Can you work these out from the model? Positions are in its coordinate system, mm. A direction names the side the tool comes from. Round coordinates to 2 decimals unless told otherwise and drop trailing zeros. Loops run counter-clockwise (first coordinate to the right, second up) from the corner with the lowest first, then second, coordinate; pieces in that order, holes last. Notation, with made-up numbers: (-34, 26.5) -> (25, 26.5) arc R33 cw to (25, 62.5) -> close; hole circle Ø5 at (28, -38). An arc over 180 degrees is marked (long way). Answer as a JSON object with one key per item and string values.
```python
from build123d import *

# Parameters (mm, degrees)
SKETCH2_W           = 23
SKETCH2_H           = 32
SKETCH2_R           = 5.5
SKETCH2_R_2         = 20
SKETCH2_W_2         = 18
SKETCH2_H_2         = 25
BOSS_EXTRUDE1_DEPTH = 3
BOSS_EXTRUDE2_DEPTH = 3
SKETCH4_W           = 180
SKETCH4_H           = 158
BOSS_EXTRUDE3_DEPTH = 3
SKETCH6_W           = 1.5
SKETCH6_H           = 3
CUT_EXTRUDE4_DEPTH  = 177
SKETCH8_W           = 180
SKETCH8_H           = 147
BOSS_EXTRUDE5_DEPTH = 3
SKETCH9_R           = 5
SKETCH9_W           = 13.5
SKETCH9_H           = 6
CUT_EXTRUDE5_DEPTH  = 10


with BuildPart() as part:
    # Sketch2 → Boss-Extrude1 (new body)
    # profile 1 of 2: a face of its own
    with BuildSketch(Plane.XY):
        Polygon((90, 180), (0, 180), (0, 130), (0, 0), (90, 0), (90, 73), (47.5, 73), (47.5, 130), (90, 130), align=None)
        with Locations((36, 37)):
            Rectangle(SKETCH2_W, SKETCH2_H, mode=Mode.SUBTRACT)
        with Locations((22, 101.5)):
            Circle(SKETCH2_R, mode=Mode.SUBTRACT)
    # profile 2 of 2: a face of its own
    with BuildSketch(Plane.XY):
        Polygon((180, 180), (90, 180), (90, 130), (132.5, 130), (132.5, 73), (90, 73), (90, 0), (180, 0), align=None)
        with Locations((142, 37)):
            Circle(SKETCH2_R_2, mode=Mode.SUBTRACT)
        with Locations((161.5, 101.5)):
            Rectangle(SKETCH2_W_2, SKETCH2_H_2, mode=Mode.SUBTRACT)
    extrude(amount=-BOSS_EXTRUDE1_DEPTH)

    # Sketch3 → Boss-Extrude2 (add)
    with BuildSketch(Plane(origin=(0, 0, 0), x_dir=(0, 0, -1), z_dir=(1, 0, 0))):
        Polygon((158, 180), (3, 180), (3, 90), (3, 0), (50, 0), (158, 0), align=None)
    boss_extrude2 = extrude(amount=BOSS_EXTRUDE2_DEPTH)

    # Mirror1: Boss-Extrude2 across plane
    add(boss_extrude2.mirror(Plane(origin=(90, 0, 0), x_dir=(0, 0, 1), z_dir=(1, 0, 0))))

    # Sketch4 → Boss-Extrude3 (add)
    with BuildSketch(Plane(origin=(0, 0, 0), x_dir=(1, 0, 0), z_dir=(0, 1, 0))):
        with Locations((90, 79)):
            Rectangle(SKETCH4_W, SKETCH4_H)
    extrude(amount=BOSS_EXTRUDE3_DEPTH)

    # Sketch6 → Cut-Extrude4 (cut)
    with BuildSketch(Plane(origin=(0, 180, 0), x_dir=(1, 0, 0), z_dir=(0, 1, 0))):
        with Locations((2.25, 151.5)):
            Rectangle(SKETCH6_W, SKETCH6_H)
    cut_extrude4 = extrude(amount=-CUT_EXTRUDE4_DEPTH, mode=Mode.SUBTRACT)

    # Mirror2: Cut-Extrude4 across plane
    add(cut_extrude4.mirror(Plane(origin=(90, 0, 0), x_dir=(0, 0, 1), z_dir=(1, 0, 0))), mode=Mode.SUBTRACT)

    # Sketch8 → Boss-Extrude5 (add)
    with BuildSketch(Plane(origin=(0, 180, 0), x_dir=(1, 0, 0), z_dir=(0, 1, 0))):
        with Locations((90, 73.5)):
            Rectangle(SKETCH8_W, SKETCH8_H)
    extrude(amount=-BOSS_EXTRUDE5_DEPTH)

    # Sketch9 → Cut-Extrude5 (cut)
    with BuildSketch(Plane(origin=(180, 0, 0), x_dir=(0, 0, -1), z_dir=(1, 0, 0))):
        with Locations((77.5, 141.3)):
            Circle(SKETCH9_R)
        with Locations((77.5, 12)):
            Rectangle(SKETCH9_W, SKETCH9_H)
    extrude(amount=-CUT_EXTRUDE5_DEPTH, mode=Mode.SUBTRACT)


solid = part.part
```
Q1. On a 3-axis mill with a long thin cutter (end or side, diameter ignored), from which of +Z, -Z, +X, -X, +Y, -Y can I reach the whole of each face in a straight line? I mean faces 1 (the flat face through (3, 93, -155)), 2 (the cylindrical face through (178.521, 136.864, -79.807)), 3 (the flat face through (91, 0, -78)), 4 (the flat face through (180, 91, -78)), 5 (the flat face through (177, 93, -75)). Say none if no direction works.
Determined:
{"face 1": "-Z, +Y", "face 2": "+X", "face 3": "+Z, -Z, +X, -X, -Y", "face 4": "+Z, -Z, +X, +Y, -Y", "face 5": "-Z"}
Q2. If I drill on L1, parallel to Y at x = 178, z = -77; L2, parallel to Y at x = 55.5, z = -128, over which ranges is the centre line in solid material (lowest first)? Write a range as [from, to].
Determined:
{"L1": "[0, 9], [15, 136.33], [146.27, 180]", "L2": "[0, 3], [177, 180]"}
Q3. I want a section at A-A, the plane y = 141.3. Write out the boundary of the cut face in (x, z), then the cut area to 3 significant figures.
Determined:
{"outline": "(0, -158) -> (3, -158) -> (3, -153) -> (1.5, -153) -> (1.5, -150) -> (3, -150) -> (3, -3) -> (177, -3) -> (177, -72.5) -> (180, -72.5) -> (180, 0) -> (0, 0) -> close; (177, -158) -> (180, -158) -> (180, -82.5) -> (177, -82.5) -> (177, -150) -> (178.5, -150) -> (178.5, -153) -> (177, -153) -> close", "area": "1,430 mm²"}
Q4. I want a section at C-C, the plane y = 37. Write out the boundary of the cut face in (x, z), then the cut area to 3 significant figures.
Determined:
{"outline": "(0, -158) -> (3, -158) -> (3, -153) -> (1.5, -153) -> (1.5, -150) -> (3, -150) -> (3, -3) -> (24.5, -3) -> (24.5, 0) -> (0, 0) -> close; (47.5, -3) -> (122, -3) -> (122, 0) -> (47.5, 0) -> close; (162, -3) -> (177, -3) -> (177, -150) -> (178.5, -150) -> (178.5, -153) -> (177, -153) -> (177, -158) -> (180, -158) -> (180, 0) -> (162, 0) -> close", "area": "1,270 mm²"}
Q5. I want a section at B-B, the plane x = 142. Write out the boundary of the cut face in (y, z).
Determined:
{"outline": "(0, -158) -> (3, -158) -> (3, -3) -> (17, -3) -> (17, 0) -> (0, 0) -> close; (57, -3) -> (177, -3) -> (177, -147) -> (180, -147) -> (180, 0) -> (57, 0) -> close"}
Q6. I want a section at D-D, the plane z = -77.5. Write out the boundary of the cut face in (x, y), then the cut area to 3 significant figures.
Determined:
{"outline": "(0, 0) -> (180, 0) -> (180, 9) -> (177, 9) -> (177, 3) -> (3, 3) -> (3, 177) -> (177, 177) -> (177, 146.3) -> (180, 146.3) -> (180, 180) -> (0, 180) -> close; (177, 15) -> (180, 15) -> (180, 136.3) -> (177, 136.3) -> close", "area": "2,080 mm²"}
Q7. We'd pull the mould along X, two halves only. Please class faces 6 (the flat face through (89, 71, 0)), 7 (the flat face through (0, 91, -78)), 8 (the flat face through (89, 3, -82)), 9 (the cylindrical face through (122.02, 37.88, -1.48)): pulls with the +X half, pulls with the -X half, needs draft (parallel to the pull), parting line crosses it, or undercut.
Determined:
{"face 6": "needs draft", "face 7": "pulls with the -X half", "face 8": "undercut", "face 9": "undercut"}
Q8. I'm going to push flat-ended pins straight in: pin 1 (14.5 mm diameter, centred on x = 22, y = 101.5, fed in from -Z); pin 2 (0.9 mm diameter, centred on x = 92, y = 178, fed in from -Z). Where does each tip first touch, or does it pass through?
Determined:
{"pin 1": "z = -3", "pin 2": "z = -147"}
